Can you work these out from the model? Positions are in its coordinate system, mm. Face numbers are marked on the shaded views. Coordinates: 2 decimals unless noted, no trailing zeros. Order: outer loops, then holes, each group sorted by start corner. A loop starts at its lowest first (then second) coordinate and runs counter-clockwise, first axis right, second up. Notation, with made-up numbers: (34, -3.75) -> (46, -3.75) arc R12 ccw to (46, 19.25) -> close; hole circle Ø1 at (53, 83). An arc over 180 degrees is marked (long way). Answer in a Markdown table with one row per item.
Autodesk Fusion 360 part; units mm, degrees
sketch "Sketch1" plane through (0, 0, 0) normal (0, 0, 1) x (1, 0, 0)
  circle A0 centre (0, 0) radius 44.5
  circle A1 centre (0, 0) radius 42.5
  dimension "d1" = 89
  dimension "d2" = 2
extrude "Extrude1" add sketch "Sketch1" against normal blind 2 contours A0 | A1 makes body 1
extrude "Extrude2" add sketch "Sketch1" along normal blind 45 bodies 1
sketch "Sketch2" plane through (0, 0, 45) normal (0, 0, 1) x (-1, 0, 0)
  circle A0 centre (0, 0) radius 42.5
  circle A1 centre (0, 0) radius 44.5
  circle A2 centre (0, 0) radius 44.5
  dimension "d7" = 89
extrude "Extrude3" add sketch "Sketch2" along normal blind 2 separate body contours A0 | A1 A2 makes body 2
sketch "Sketch3" plane through (0, 0, 47) normal (0, 0, 1) x (-1, 0, 0)
  circle A0 centre (0, 0) radius 44.5
  circle A1 centre (0, -38) radius 2.5
  circle A2 centre (0, -38) radius 4
  dimension "d10" = 5
  dimension "d12" = 1.5
  dimension "d24" = 38
extrude "Extrude4" add sketch "Sketch3" against normal blind 3.5 contours A1 | A2 bodies 2
extrude "Extrude5" cut sketch "Sketch3" against normal blind 2 contours A1 bodies 2
pattern_circular "C-Pattern1" count 11 over 360 about axis through (0, 0, 1.75) along (0, 0, 1) of "Extrude4", "Extrude5"
sketch "Sketch5" plane through (0, 0, 47) normal (0, 0, 1) x (-1, 0, 0)
  circle A0 centre (10.7058, 36.4607) radius 2.5
  circle A1 centre (28.7185, 24.8847) radius 2.5
  circle A2 centre (37.6132, 5.408) radius 2.5
  circle A3 centre (34.566, -15.7858) radius 2.5
  circle A4 centre (20.5444, -31.9676) radius 2.5
  circle A5 centre (0, -38) radius 2.5
  circle A6 centre (0, 0) radius 44.5
  circle A7 centre (0, 0) radius 34
  circle A8 centre (0, -38) radius 4
  circle A9 centre (-37.6132, 5.408) radius 2.5
  circle A10 centre (-28.7185, 24.8847) radius 2.5
  circle A11 centre (-10.7058, 36.4607) radius 2.5
  circle A12 centre (-34.566, -15.7858) radius 2.5
  circle A13 centre (-20.5444, -31.9676) radius 2.5
extrude "Extrude6" cut sketch "Sketch5" against normal blind 5 contours A7 bodies 2
sketch "Sketch7" plane through (0, 0, 47) normal (0, 0, 1) x (-1, 0, 0)
  circle A0 centre (0, 0) radius 34
  circle A1 centre (10.7058, 36.4607) radius 2.5
  circle A2 centre (28.7185, 24.8847) radius 2.5
  circle A3 centre (37.6132, 5.408) radius 2.5
  circle A4 centre (34.566, -15.7858) radius 2.5
  circle A5 centre (20.5444, -31.9676) radius 2.5
  circle A6 centre (0, -38) radius 2.5
  circle A7 centre (0, 0) radius 44.5
  arc A8 (41.3317, -9.8965) -> (42.4456, -2.1489) centre (0, 0) ccw
  arc A9 (34.5241, -8.2665) -> (41.3317, -9.8965) centre (37.9279, -9.0815) ccw
  arc A10 (34.5241, -8.2665) -> (35.4546, -1.795) centre (0, 0) ccw
  arc A11 (42.4456, -2.1489) -> (35.4546, -1.795) centre (38.9501, -1.9719) ccw
  arc A12 (37.9279, -9.0815) -> (38.9501, -1.9719) centre (0, 0) ccw construction
  circle A13 centre (-37.6132, 5.408) radius 2.5
  circle A14 centre (-28.7185, 24.8847) radius 2.5
  circle A15 centre (-10.7058, 36.4607) radius 2.5
  circle A16 centre (-34.566, -15.7858) radius 2.5
  circle A17 centre (34.566, -15.7858) radius 4
  circle A18 centre (37.6132, 5.408) radius 4
  circle A19 centre (-20.5444, -31.9676) radius 2.5
  dimension "d25" = 2
  dimension "d26" = 39
combine "Combine1" operation add target body 1 tool bodies 2
sketch "Sketch9" plane through (0, 0, 47) normal (0, 0, 1) x (-1, 0, 0)
  circle A0 centre (0, 0) radius 44.5 construction
  line L0 (0, 0) -> (-7.973, -43.7799)
  line L1 (0, 0) -> (-36.5115, -25.4393)
  circle A1 centre (0, 0) radius 34 construction
  circle A2 centre (0, 0) radius 42.5
  circle A3 centre (28.7185, 24.8847) radius 4
  circle A4 centre (10.7058, 36.4607) radius 4
extrude "Extrude8" cut sketch "Sketch9" against normal blind 6 contours L0 L1 A2 picked at (-13.7041, -24.73) bodies 1
fillet "Fillet1" radius 4 2 edges at (6.0917, 33.4498, 46) (27.8964, 19.4368, 46) on bodies 1
fillet "Fillet2" radius 3 2 edges at (7.6146, 41.8123, 46) (34.8706, 24.296, 46) on bodies 1
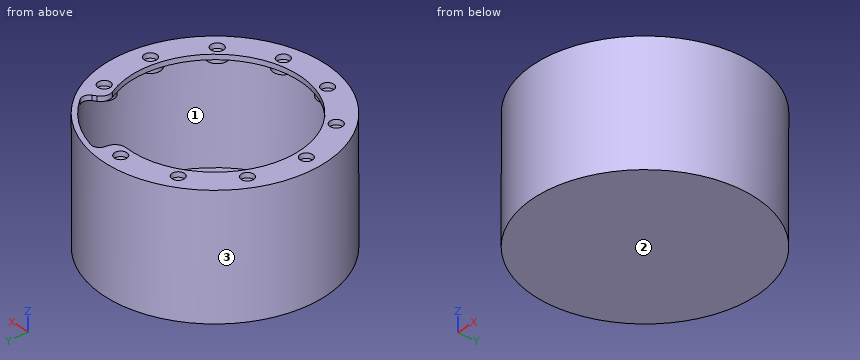
(1) I need wall thicknesses on line 1 (Y direction, x = 0, z = 46.3); line 2 (Z direction, x = 32, y = 14.5); line 3 (Z direction, x = 21.5, y = -31). Which ranges of each line are inside material? Lowest first, please. Write a range as [from, to].
Response values:
| item | result |
|---|---|
| line 1 | [-44.5, -34], [34, 35.5], [40.5, 44.5] |
| line 2 | [-2, 0], [43.5, 47] |
| line 3 | [-2, 0], [45, 47] |
(2) Suppose I cut it at B-B (y = -18.5). Please give me the cut outline in (x, z), and give its area (3 significant figures).
Response values:
| item | result |
|---|---|
| outline | (-40.47, -2) -> (40.47, -2) -> (40.47, 47) -> (28.53, 47) -> (28.53, 45) -> (38.26, 45) -> (38.26, 0) -> (-38.26, 0) -> (-38.26, 45) -> (-28.53, 45) -> (-28.53, 47) -> (-40.47, 47) -> close |
| area | 409 mm2 |
(3) Will these pins go through, and if not, where does the flat tip stop? pin 1 Ø8 at (x, y) = (-10.71, -36.46) entering from +Z; pin 2 Ø12 at (y, z) = (28, 27.5) entering from +X; pin 3 Ø4 at (y, z) = (-23.5, 3.5) entering from +X; pin 4 Ø2 at (x, z) = (-15.5, 30) entering from -Y.
Response values:
| item | result |
|---|---|
| pin 1 | z = 47 |
| pin 2 | x = 38.68 |
| pin 3 | x = 38.96 |
| pin 4 | y = -42.07 |
(4) We'd pull the mould along Y, two halves only. Please class the marked faces 1, 2 and 3: +Y half, -Y half, draft (parallel to the pull), parting line (faces both ways), or undercut.
Response values:
| item | result |
|---|---|
| face 1 | undercut |
| face 2 | draft |
| face 3 | parting line |
(5) Suppose I cut it at A-A (z = 6.5). Please give me the cut outline in (x, y).
Response values:
| item | result |
|---|---|
| outline | circle Ø89 at (0, 0); hole circle Ø85 at (0, 0) |
